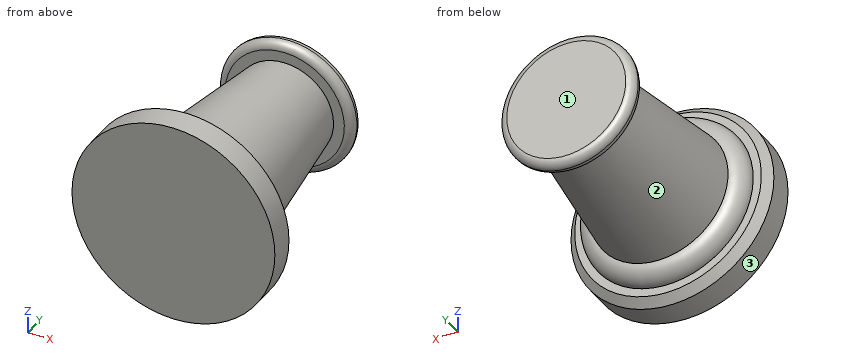
from build123d import *

# Parameters (mm, degrees)
CHAMFER1_SIZE = 0.762
FILLET2_R     = 1.524
FILLET3_R     = 0.762


with BuildPart() as part:
    # Sketch3 → Revolve1 (revolve)
    with BuildSketch(Plane.XY, mode=Mode.PRIVATE) as revolve1_sk:
        Polygon((0, 0), (-9.525, 0), (-9.525, 3.175), (-8.001, 3.175), (-8.001, 4.699), (-6.477, 4.699), (-4.572, 19.05), (-6.35, 19.05), (-6.35, 20.574), (0, 20.574), align=None)
    revolve(revolve1_sk.sketch.rotate(Axis((0, 20.574, 0), (0, -1, 0)), 270), axis=Axis((0, 20.574, 0), (0, -1, 0)))

    # Chamfer1
    chamfer1_edges = [part.edges().sort_by_distance(p)[0] for p in [
        (0, 3.175, -9.525),
    ]]
    chamfer(chamfer1_edges, length=CHAMFER1_SIZE)

    # Fillet2
    fillet2_edges = [part.edges().sort_by_distance(p)[0] for p in [
        (0, 4.699, -8.001),
    ]]
    fillet(fillet2_edges, radius=FILLET2_R - 0.0001)  # a hair under: the kernel refuses the full size

    # Fillet3
    fillet3_edges = [part.edges().sort_by_distance(p)[0] for p in [
        (0, 20.574, -6.35),
        (0, 19.05, -6.35),
    ]]
    fillet(fillet3_edges, radius=FILLET3_R - 0.0001)  # a hair under: the kernel refuses the full size


solid = part.part
Verification items for the finished model (mm, model axes). Face numbers are marked on the shaded views. Round coordinates to 2 decimals unless told otherwise and drop trailing zeros. Loops run counter-clockwise (first coordinate to the right, second up) from the corner with the lowest first, then second, coordinate; pieces in that order, holes last. Notation, with made-up numbers: (-10, 23) - (20, 23) arc R24 cw to (20, 55) - close; hole circle Ø9 at (23.25, 46). An arc over 180 degrees is marked (long way). Use one line per item in the form item = value.
1. Gauge pin test, flat ends, axial feed: pin 1 Ø10 at (x, y) = (6, 18) entering from -Z; pin 2 Ø6 at (x, y) = (-1.5, 5.5) entering from +Z; pin 3 Ø6 at (x, y) = (6.5, 5.5) entering from +Z. Record the tip position at first contact, or that the pin passes through.
A:
pin_1 = -6.21
pin_2 = 9.35
pin_3 = 7.53
2. Draft check along Y on the marked faces 1, 2 and 3. Enter one of: pulls with the +Y half, pulls with the -Y half, needs draft (parallel to the pull), parting line crosses it, or undercut.
A:
face_1 = pulls with the +Y half
face_2 = undercut
face_3 = needs draft
3. Scan lines: probe 1 along Y at (x, z) = (2, -6.25); probe 2 along Z at (x, y) = (-1.25, 17.5); probe 3 along X at (y, z) = (4, 0.5). Record each from-to range of solid material in increasing order.
A:
probe_1 = 0 to 4.7
probe_2 = -4.61 to 4.61
probe_3 = -7.74 to 7.74
4. Section check C-C on y = 13. Record the cut outline in (x, z), and give its area (3 significant figures).
A:
outline = circle Ø10.75 at (0, 0)
area = 90.8 mm²
5. Section check D-D on y = 6.75. Record the cut outline in (x, z), and give its area (3 significant figures).
A:
outline = circle Ø12.41 at (0, 0)
area = 121 mm²
